from build123d import *

# Parameters (mm, degrees)
SKETCH1_W               = 7.5
SKETCH1_H               = 3.5
SKETCH8_R               = 1.75
CUT_EXTRUDE6_DEPTH      = 10
CUT_EXTRUDE7_DEPTH      = 9.986100378
CUT_EXTRUDE7_DEPTH_BACK = 9.986100378
SKETCH9_R               = 0.79375


with BuildPart() as part:
    # Sketch1 → Revolve1 (revolve)
    with BuildSketch(Plane.XY, mode=Mode.PRIVATE) as revolve1_sk:
        with Locations((3.75, 1.75)):
            Rectangle(SKETCH1_W, SKETCH1_H)
    revolve(revolve1_sk.sketch.rotate(Axis((-11.701807229, 0, 0), (1, 0, 0)), 90), axis=Axis((-11.701807229, 0, 0), (1, 0, 0)))

    # Sketch8 → Cut-Extrude6 (cut)
    with BuildSketch(Plane.ZY):
        Circle(SKETCH8_R)
    extrude(amount=-CUT_EXTRUDE6_DEPTH, mode=Mode.SUBTRACT)

    # Sketch9 → Cut-Extrude7 (cut, two sides: drawn at the far end of the back side and taken through both)
    with BuildSketch(Plane.XY.offset(-CUT_EXTRUDE7_DEPTH_BACK)):
        with Locations((5.5, 0)):
            Circle(SKETCH9_R)
    extrude(amount=CUT_EXTRUDE7_DEPTH + CUT_EXTRUDE7_DEPTH_BACK, mode=Mode.SUBTRACT)


solid = part.part
Design review of the part built by this model. Coordinates are the model's own, in mm. Round coordinates to 2 decimals unless told otherwise and drop trailing zeros. Write each loop counter-clockwise with the first axis right and the second up, starting at its lowest first coordinate (ties: lowest second). Pieces come first, ordered by that corner, then holes. Notation, with made-up numbers: (25.25, -27.75) - (49.25, -27.75) arc R19 ccw to (49.25, 4.25) - close; hole circle Ø10 at (53, -23.5). An arc over 180 degrees is marked (long way). Return JSON: item names as keys, results as strings. Group by question number.
Item 1: For probe 1 along Y at (x, z) = (3, 0); probe 2 along X at (y, z) = (0, -2.05); probe 3 along Z at (x, y) = (6.5, -0.75), list the stretches that pass through material, from the lowest coordinate up. Write a range as [from, to].
Item 2: We need section D-D on z = 2.75. Write out the cut boundary in (x, y), and give its area (3 significant figures).
Item 3: The part is to be moulded in two halves that separate along Y. For faces 1 (the face through (7.5, 1, 2)), 2 (the face through (3.8, -1.05, 3.34)), 3 (the face through (5.397, 0.787, -2.544)), say which applies: pulls with the +Y half, pulls with the -Y half, needs draft (parallel to the pull), parting line crosses it, or undercut.
Item 4: We need section C-C on x = 5.5. Write out the cut boundary in (y, z).
Item 5: Insertion check: P1, Ø3, axis at x = 6.5, z = -2.5, coming from the -Y side; P2, Ø1, axis at x = 3, y = 2.5, coming from the -Z side. Each pin has a flat end and moves straight along its axis. Give the tip position at first contact, or say it passes through.
Item 6: We need section B-B on z = 0. Write out the cut boundary in (x, y), and give its area (4 significant figures).
Item 7: We need section A-A on y = 0. Write out the cut boundary in (x, z), and give its area (3 significant figures).
Model answer:
{
 "1": {"probe 1": "y = [-3.5, -1.75], [1.75, 3.5]", "probe 2": "x = [0, 4.71], [6.29, 7.5]", "probe 3": "z = [-3.42, -1.58], [1.58, 3.42]"},
 "2": {"outline": "(0, -2.17) - (7.5, -2.17) - (7.5, 2.17) - (0, 2.17) - close; hole circle Ø1.59 at (5.5, 0)", "area": "30.5 mm²"},
 "3": {"face 1": "needs draft", "face 2": "parting line crosses it", "face 3": "undercut"},
 "4": {"outline": "(-0.79, -3.41) - (-0.79, -1.56) arc R1.75 cw to (-0.79, 1.56) - (-0.79, 3.41) arc R3.5 ccw to start; (0.79, -3.41) arc R3.5 ccw to (0.79, 3.41) - (0.79, 1.56) arc R1.75 cw to (0.79, -1.56) - close"},
 "5": {"P1": "stops at y = -3.35", "P2": "stops at z = -2.87"},
 "6": {"outline": "(0, -3.5) - (7.5, -3.5) - (7.5, -1.75) - (0, -1.75) - close; (0, 1.75) - (7.5, 1.75) - (7.5, 3.5) - (0, 3.5) - close", "area": "26.25 mm²"},
 "7": {"outline": "(0, -3.5) - (4.71, -3.5) - (4.71, -1.75) - (0, -1.75) - close; (0, 1.75) - (4.71, 1.75) - (4.71, 3.5) - (0, 3.5) - close; (6.29, -3.5) - (7.5, -3.5) - (7.5, -1.75) - (6.29, -1.75) - close; (6.29, 1.75) - (7.5, 1.75) - (7.5, 3.5) - (6.29, 3.5) - close", "area": "20.7 mm²"}
}
